from build123d import *

# Parameters (mm, degrees)
F0_W     = 128.6668404937
F0_H     = 100.6218641996
F0_R     = 25.0442711875
F1_DEPTH = 50.8


# Not quite as in the source:
# - the program builds the solid bodies; features that only make, move or delete a surface that nothing else refers to are left out


with BuildPart() as f1:
    # F0 (on Front) → F1 (new body)
    with BuildSketch(Plane.XZ):
        with Locations((-1.2895353138, -2.8847418725)):
            Rectangle(F0_W, F0_H)
        Circle(F0_R, mode=Mode.SUBTRACT)
    extrude(amount=F1_DEPTH)


solid = f1.part
Part model, mm, in its own coordinate system. Coordinates: 2 decimals unless noted, no trailing zeros. Order: outer loops, then holes, each group sorted by start corner. A loop starts at its lowest first (then second) coordinate and runs counter-clockwise, first axis right, second up.
(1) Pull direction Z, two halves, no side cores. Call faces 1 (the face through (-5.43, -25.04, -24.45)), 2 (the face through (-2, -25, -53.196)), 3 (the face through (-16, 0, -25)): pulls with the +Z half, pulls with the -Z half, needs draft (parallel to the pull), parting line crosses it, or undercut.
Check sheet entries:
face 1: undercut
face 2: pulls with the -Z half
face 3: needs draft
(2) Probe L1, parallel to Z at x = 0, y = -25.5; L2, parallel to Z at x = -16, y = -47; L3, parallel to X at y = -23.5, z = 10. List the from-to ranges inside material, lowest first.
Check sheet entries:
L1: z = -53.2 to -25.04, 25.04 to 47.43
L2: z = -53.2 to -19.27, 19.27 to 47.43
L3: x = -65.62 to -22.96, 22.96 to 63.04
(3) Slice it at A-A, the plane x = 0. Write the cut outline in (y, z).
Check sheet entries:
outline: (-50.8, -53.2) - (0, -53.2) - (0, -25.04) - (-50.8, -25.04) - close; (-50.8, 25.04) - (0, 25.04) - (0, 47.43) - (-50.8, 47.43) - close
(4) Slice it at B-B, the plane z = 0. Write the cut outline in (x, y), and give its area (3 significant figures).
Check sheet entries:
outline: (-65.62, -50.8) - (-25.04, -50.8) - (-25.04, 0) - (-65.62, 0) - close; (25.04, -50.8) - (63.04, -50.8) - (63.04, 0) - (25.04, 0) - close
area: 3,990 mm2
(5) Slice it at C-C, the plane y = -37.5. Write the cut outline in (x, z).
Check sheet entries:
outline: (-65.62, -53.2) - (63.04, -53.2) - (63.04, 47.43) - (-65.62, 47.43) - close; hole circle Ø50.09 at (0, 0)
